from build123d import *

# Parameters (mm, degrees)
BASE_SKETCH_W      = 15
BASE_SKETCH_H      = 15
BASE_DEPTH         = 15
NUT_HOLE_SKETCH_R  = 2.45
NUT_HOLE_DEPTH     = 10
ROUNDING_R         = 6
THUMB_HOLE_DEPTH   = 23.5
KRUHOV_POLE1_COUNT = 2


with BuildPart() as part:
    # Base sketch → Base (new body)
    with BuildSketch(Plane.XY):
        Rectangle(BASE_SKETCH_W, BASE_SKETCH_H)
    extrude(amount=BASE_DEPTH)

    # Nut hole sketch → Nut hole (cut)
    with BuildSketch(Plane.XY.offset(15)):
        Circle(NUT_HOLE_SKETCH_R)
    extrude(amount=-NUT_HOLE_DEPTH, mode=Mode.SUBTRACT)

    # Rounding
    rounding_edges = [part.edges().sort_by_distance(p)[0] for p in [
        (7.5, -7.5, 7.5),
        (-7.5, -7.5, 7.5),
        (-7.5, 7.5, 7.5),
        (7.5, 7.5, 7.5),
    ]]
    fillet(rounding_edges, radius=ROUNDING_R)

    # Thumb hole sketch → Thumb hole (cut, through all)
    with BuildSketch(Plane.XZ.offset(7.5)):
        with BuildLine():
            Line((-7.5, 13), (-7.5, 2))
            ThreePointArc((-7.5, 2), (-5.5, 7.5), (-7.5, 13))
        make_face()
    thumb_hole = extrude(amount=-THUMB_HOLE_DEPTH, mode=Mode.SUBTRACT)

    # Kruhové pole1: Thumb hole ×2 about axis
    kruhov_pole1_axis = Axis((0, 0, 7.5), (0, 1, 0))
    for i in range(1, KRUHOV_POLE1_COUNT):
        add(thumb_hole.rotate(kruhov_pole1_axis, i * 360 / KRUHOV_POLE1_COUNT), mode=Mode.SUBTRACT)


solid = part.part
Geometry check sheet. Reference: the model listing, model coordinates, mm. A direction names the side the tool comes from. Round coordinates to 2 decimals unless told otherwise and drop trailing zeros. Order: outer loops, then holes, each group sorted by start corner. A loop starts at its lowest first (then second) coordinate and runs counter-clockwise, first axis right, second up. Notation, with made-up numbers: (26, 40) - (46, 40) arc R29 cw to (46, 74) - close; hole circle Ø10 at (32.5, 39.5). An arc over 180 degrees is marked (long way). One line per question, with ' | ' between items. Start each with the question number.
(1) Sectioned sample at C-C on x = 0. Record the cut outline in (y, z).
(2) Release check for a two-part mould opening along X. For faces 1 (the flat face through (-7.5, 0, 14)), 2 (the flat face through (0, 0, 5)), 3 (the flat face through (0, 7.5, 7)) record: released by +X, released by -X, zero draft, split by the parting line, or undercut.
(3) Access from +Z, -Z, +X, -X, +Y, -Y to the whole of each face (thin tool, end or side, straight path). Record for faces 4 (the cylindrical face through (4.89, -6.45, 7.6)), 5 (the cylindrical face through (-0.5, -2.4, 10.1)).
(4) Depth check by flat-ended pin: pin 1 Ø4 at (y, z) = (-1, 10.5) entering from -X; pin 2 Ø2 at (y, z) = (-5.5, 10.5) entering from +X; pin 3 Ø1 at (x, z) = (-4, 2) entering from +Y. Enter the tip coordinate at first touch or a pass-through.
(5) Sectioned sample at D-D on z = 6.25. Record the cut outline in (x, y), and give its area (3 significant figures).
(6) Sectioned sample at A-A on x = -6.25. Record the cut outline in (y, z), and give its area (3 significant figures).
(7) Thickness scan on L1, parallel to Y at x = 0, z = 10.25; L2, parallel to X at y = -2.75, z = 7.25; L3, parallel to Z at x = 6.75, y = 1. Record the ranges inside material, lowest first. Write a range as [from, to].
Conclusion:
1) outline: (-7.5, 0) - (7.5, 0) - (7.5, 15) - (2.45, 15) - (2.45, 5) - (-2.45, 5) - (-2.45, 15) - (-7.5, 15) - close
2) face 1: released by -X | face 2: undercut | face 3: zero draft
3) face 4: +Z, -Z, +X, -Y | face 5: +Z
4) pin 1: stops at x = -7.11 | pin 2: stops at x = 6.41 | pin 3: stops at y = 7.16
5) outline: (-5.59, -5.89) arc R6 ccw to (-1.5, -7.5) - (1.5, -7.5) arc R6 ccw to (5.59, -5.89) - (5.59, 5.89) arc R6 ccw to (1.5, 7.5) - (-1.5, 7.5) arc R6 ccw to (-5.59, 5.89) - close; hole circle Ø4.9 at (0, 0) | area: 141 mm2
6) outline: (-5.17, 0) - (5.17, 0) - (5.17, 4) - (-5.17, 4) - close; (-5.17, 11) - (5.17, 11) - (5.17, 15) - (-5.17, 15) - close | area: 82.6 mm2
7) L1: y = [-7.5, -2.45], [2.45, 7.5] | L2: x = [-5.5, 5.5] | L3: z = [0, 3.05], [11.95, 15]
